Design review of the part built by this model. Coordinates are the model's own, in mm. Face numbers are marked on the shaded views. A direction names the side the tool comes from. Coordinates: 2 decimals unless noted, no trailing zeros. Order: outer loops, then holes, each group sorted by start corner. A loop starts at its lowest first (then second) coordinate and runs counter-clockwise, first axis right, second up. Notation, with made-up numbers: (72.25, 81.5) - (85.25, 81.5) arc R18 ccw to (85.25, 100.5) - close; hole circle Ø1 at (-23, -6.75). An arc over 180 degrees is marked (long way). Write item = value, one per line. Start each with the question number.
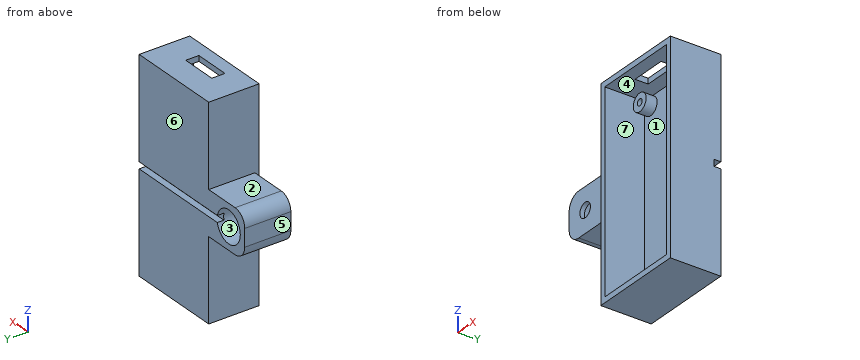
Autodesk Inventor part; units mm, degrees
ref_plane "YZ Plane" through (0, 0, 0) normal (1, 0, 0) x (0, 1, 0)
ref_plane "XZ Plane" through (0, 0, 0) normal (0, 1, 0) x (-1, 0, 0)
ref_plane "XY Plane" through (0, 0, 0) normal (0, 0, 1) x (1, 0, 0)
sketch "Sketch1" plane through (0, 0, 0) normal (0, 1, 0) x (-1, 0, 0)
  line L0 (-7.5, 22.32) -> (-26.74, 22.32)
  line L1 (-26.74, 22.32) -> (-26.74, -22.32)
  line L2 (-26.74, -22.32) -> (-7.5, -22.32)
  line L3 (-7.5, -22.32) -> (-7.5, 22.32)
  line L4 (-7.5, 5) -> (2, 5)
  line L5 (5, 2) -> (5, -2)
  line L6 (2, -5) -> (-7.5, -5)
  line L7 (-7.5, -5) -> (-7.5, 5)
  line L8 (0, 0.75) -> (-7.5, 0.75)
  line L9 (-7.5, 0.75) -> (-7.5, -0.75)
  line L10 (-7.5, -0.75) -> (0, -0.75)
  line L11 (0, -0.75) -> (0, 0.75)
  circle A0 centre (0, 0) radius 3.625
  arc A1 (5, 2) -> (2, 5) centre (2, 2) ccw
  arc A2 (2, -5) -> (5, -2) centre (2, -2) ccw
  circle A3 centre (0, 0) radius 1.65
  line L12 (-9.5, 20.32) -> (-24.74, 20.32) construction
  line L13 (-24.74, 20.32) -> (-24.74, -20.32) construction
  line L14 (-24.74, -20.32) -> (-9.5, -20.32) construction
  line L15 (-9.5, -20.32) -> (-9.5, 20.32) construction
  circle A4 centre (-9.5, 20.32) radius 2
  circle A5 centre (-9.5, 20.32) radius 0.75
  circle A6 centre (-9.5, -20.32) radius 2
  circle A7 centre (-9.5, -20.32) radius 0.75
  circle A8 centre (-24.74, -20.32) radius 2
  circle A9 centre (-24.74, -20.32) radius 0.75
  circle A10 centre (-24.74, 20.32) radius 2
  circle A11 centre (-24.74, 20.32) radius 0.75
  line L16 (-27.99, -23.57) -> (-6.25, -23.57)
  line L17 (-6.25, -23.57) -> (-6.25, 23.57)
  line L18 (-6.25, 23.57) -> (-27.99, 23.57)
  line L19 (-27.99, 23.57) -> (-27.99, -23.57)
  line L20 (-7.5, 0.75) -> (-27.99, 0.75)
  line L21 (-27.99, 0.75) -> (-27.99, -0.75)
  line L22 (-27.99, -0.75) -> (-7.5, -0.75)
  line L23 (-7.5, -0.75) -> (-7.5, 0.75)
  point P0 (-6.25, -5)
  point P1 (-6.25, 5)
  point P2 (-3.5466, 0.75)
  point P3 (-3.5466, -0.75)
  point P4 (-27.99, 0)
  dimension "d2" = 10
  dimension "d3" = 12.5
  dimension "d4" = 7.25
  dimension "d5" = 1.5
  dimension "d6" = 0.75
  dimension "d7" = 0
  dimension "d8" = 5
  dimension "d10" = 5
  dimension "d11" = 3
  dimension "d12" = 3.3
  dimension "d13" = 40.64
  dimension "d14" = 15.24
  dimension "d15" = 1.5
  dimension "d16" = 4
  dimension "d17" = 1.25
  dimension "d18" = 1.25
  dimension "d19" = 1.25
  dimension "d20" = 1.25
  dimension "d21" = 20.32
  dimension "d25" = 0
extrude "Extrusion1" add sketch "Sketch1" along normal blind 1.5 contours L3 A4 L0 | L0 L1 L20 L19 L18 L17 L4 L3 | A4 L3 L20 L1 A10 L0 | A4 | A10 L1 L0 | A10 | L4 L17 L8 L3 | L4 A1 L5 A2 L6 L17 L10 A0 L8 | L10 L17 L6 L3 | L3 A6 L2 A8 L1 L22 | L1 L2 L3 L6 L17 L16 L19 L22 | A8 L2 L1 | A8 | A6 | L3 L2 A6 | A5 | A7 | A9 | A11
extrude "Extrusion2" add sketch "Sketch1" against normal blind 3.5 contours A4 | A10 | A8 | A6
extrude "Extrusion3" add sketch "Sketch1" against normal blind 1 contours L3 A4 L0 | L0 L1 L20 L19 L18 L17 L4 L3 | A4 L3 L20 L1 A10 L0 | A4 | A10 L1 L0 | A10 | L4 L17 L8 L3 | L8 L17 L10 L3 | L3 L22 L1 L20 | L1 L22 L19 L20 | L10 L17 L6 L3 | L3 A6 L2 A8 L1 L22 | L1 L2 L3 L6 L17 L16 L19 L22 | A8 L2 L1 | A8 | A6 | L3 L2 A6 | A5 | A7 | A9 | A11
extrude "Extrusion4" add sketch "Sketch1" against normal blind 9 contours L4 A1 L5 A2 L6 L17 L10 A0 L8 | L8 A0 L10 L17
extrude "Extrusion5" add sketch "Sketch1" against normal blind 10 contours L0 L1 L20 L19 L18 L17 L4 L3 | L4 L17 L8 L3 | L8 L17 L10 L3 | L1 L22 L19 L20 | L10 L17 L6 L3 | L1 L2 L3 L6 L17 L16 L19 L22
sketch "Sketch2" plane through (0, -9, 0) normal (0, -1, 0) x (1, 0, 0)
  circle A0 centre (0, 0) radius 3.625
  circle A1 centre (0, 0) radius 1.65
extrude "Extrusion6" add sketch "Sketch2" against normal blind 1
sketch "Sketch3" plane through (26.74, -10, 22.32) normal (0, 0, -1) x (-1, 0, 0)
  line L0 (17.99, 6.5) -> (16.49, 6.5)
  line L1 (2.75, 6.5) -> (1.25, 6.5)
  line L2 (13.695, 2.85) -> (5.545, 2.85)
  line L3 (5.545, 2.85) -> (5.545, 5.85)
  line L4 (5.545, 5.85) -> (13.695, 5.85)
  line L5 (13.695, 5.85) -> (13.695, 2.85)
  line L6 (-1.25, 0) -> (-1.25, 11.5)
  line L7 (20.49, 0) -> (20.49, 11.5)
  point P0 (26.74, 10)
  point P1 (13.695, 4.35)
  point P2 (2, 6.5)
  dimension "d36" = 8.15
  dimension "d37" = 3
  dimension "d38" = 21.74
  dimension "d39" = 6.795
  dimension "d42" = 0.65
extrude "Extrusion7" cut sketch "Sketch3" against normal through all
equation "\"d2\" = 2 * d8"
equation "\"d18\" = d17"
equation "\"d19\" = d18"
equation "\"d20\" = d18"
properties part number "Arduino Mount"
Item 1: Add section B-B on z = 0. Give the boundary of the cut face in (x, y) (3 decimals), plus the area to 3 significant figures.
Item 2: For line 1 (X direction, y = -1.75, z = 0) (3 decimals); line 2 (X direction, y = -3.5, z = 13); line 3 (Z direction, x = 18, y = -2.5), list the stretches that pass through material, from the lowest coordinate up.
Item 3: Mouldability with a two-part tool opening along X and no side actions: class the marked faces 4, 5, 6 and 7 as +X half, -X half, draft (parallel to the pull), parting line (faces both ways), or undercut.
Item 4: For P1, Ø1.2, axis at x = 9, z = -20, coming from the -Y side; P2, Ø1.5, axis at y = -5, z = -17, coming from the -X side; P3, Ø4, axis at x = 2.5, y = -1, coming from the -Z side, all flat-tipped, find the tip position at first contact; note any pin that passes through.
Item 5: Add section D-D on y = -1.75. State how many separate pieces and enclosed holes the cut face has, plus the area to 3 significant figures.
Item 6: Add section C-C on x = 12. Give the boundary of the cut face in (y, z).
Item 7: Add section A-A on x = 18.5. Give the boundary of the cut face in (y, z).
Item 8: For the marked faces 1, 2 and 3, list the 3-axis set-ups (+Z, -Z, +X, -X, +Y, -Y) from which the entire face can be reached by the end or side of a thin tool; tool diameter is ignored.
Worked out:
q1.outline = (-5, -9) - (-1.65, -9) - (-1.65, -8) - (-3.625, -8) - (-3.625, 1.5) - (-5, 1.5) - close; (1.65, -9) - (6.25, -9) - (6.25, -10) - (7.5, -10) - (7.5, -1) - (26.74, -1) - (26.74, -10) - (27.99, -10) - (27.99, 0) - (3.625, 0) - (3.625, -8) - (1.65, -8) - close
q1.area = 86.3 mm2
q2.line_1 = -5 to -3.625, 3.625 to 7.5, 26.74 to 27.99
q2.line_2 = 6.25 to 7.5, 26.74 to 27.99
q2.line_3 = -23.57 to -22.32, 22.32 to 23.57
q3.face_4 = undercut
q3.face_5 = -X half
q3.face_6 = draft
q3.face_7 = undercut
q4.P1 = -3.5
q4.P2 = 6.25
q4.P3 = -5
q5.separate_pieces = 5
q5.enclosed_holes = 6
q5.area = 277 mm2
q6.outline = (-10, -23.57) - (1.5, -23.57) - (1.5, -0.75) - (0, -0.75) - (0, 0.75) - (1.5, 0.75) - (1.5, 23.57) - (-10, 23.57) - (-10, 22.32) - (-1, 22.32) - (-1, -22.32) - (-10, -22.32) - close
q7.outline = (-10, -23.57) - (1.5, -23.57) - (1.5, -0.75) - (0, -0.75) - (0, 0.75) - (1.5, 0.75) - (1.5, 23.57) - (-4.15, 23.57) - (-4.15, 22.32) - (-1, 22.32) - (-1, -22.32) - (-10, -22.32) - close; (-10, 22.32) - (-7.15, 22.32) - (-7.15, 23.57) - (-10, 23.57) - close
q8.face_1 = -Y
q8.face_2 = +Z, -X, +Y, -Y
q8.face_3 = +Y
